Print and shaded views of the part. All mm, measured from the part's lowest x, y and z. Coordinates: 2 decimals unless noted, no trailing zeros. Order: outer loops, then holes, each group sorted by start corner. A loop starts at its lowest first (then second) coordinate and runs counter-clockwise, first axis right, second up. Notation, with made-up numbers: (-31.75, 44) - (-19.75, 44) arc R19 cw to (-19.75, 65) - close; hole circle Ø11 at (36, 54.25). An arc over 180 degrees is marked (long way). Write each question's results on one line, items separated by ' | '.
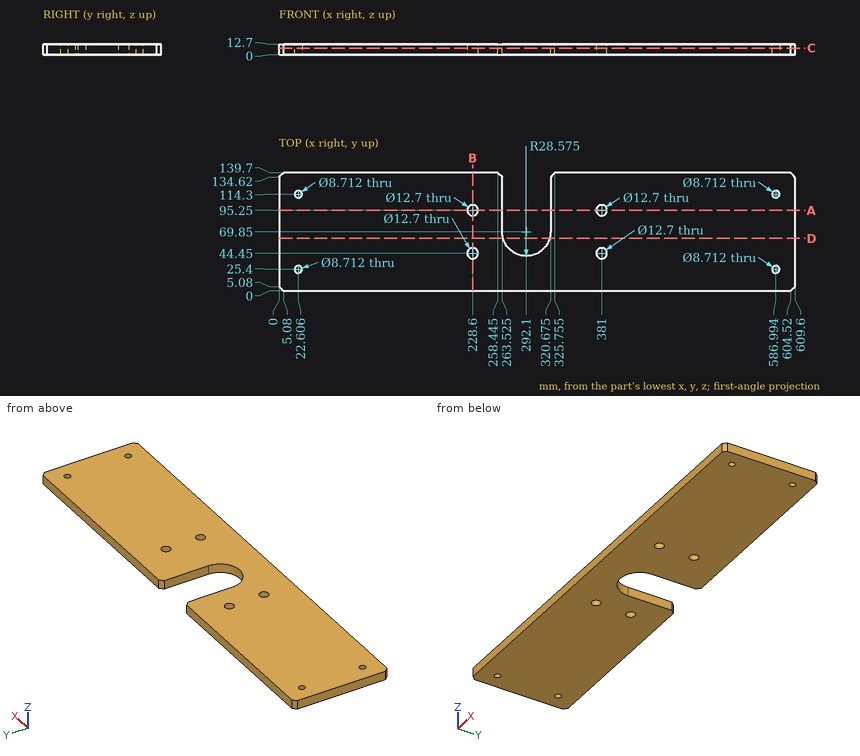
1. Band-saw the part on A-A on y = 95.25. Give the cut face in (x, z) (3 decimals), then the cut area to 3 significant figures.
Solved:
outline: (0, 0) - (222.25, 0) - (222.25, 12.7) - (0, 12.7) - close; (234.95, 0) - (263.525, 0) - (263.525, 12.7) - (234.95, 12.7) - close; (320.675, 0) - (374.65, 0) - (374.65, 12.7) - (320.675, 12.7) - close; (387.35, 0) - (609.6, 0) - (609.6, 12.7) - (387.35, 12.7) - close | area: 6,690 mm2
2. Band-saw the part on B-B on x = 228.6. Give the cut face in (y, z), then the cut area to 3 significant figures.
Solved:
outline: (0, 0) - (38.1, 0) - (38.1, 12.7) - (0, 12.7) - close; (50.8, 0) - (88.9, 0) - (88.9, 12.7) - (50.8, 12.7) - close; (101.6, 0) - (139.7, 0) - (139.7, 12.7) - (101.6, 12.7) - close | area: 1,450 mm2
3. Band-saw the part on C-C on z = 7.75. Give the number of separate pieces and of enclosed holes in the cut face, then the cut area to 3 significant figures.
Solved:
separate pieces: 1 | enclosed holes: 8 | area: 79,100 mm2
4. Drop flat-ended pins along their axis: pin 1 Ø7.5 at (x, y) = (381, 44.45) entering from -Z; pin 2 Ø1.5 at (x, z) = (307.5, 5.5) entering from +Y; pin 3 Ø3 at (x, z) = (262, 5) entering from +Y (1 decimal). Give the stop position or say it passes through.
Solved:
pin 1: passes through | pin 2: stops at y = 46.28 | pin 3: stops at y = 137.6
5. Probe line 1 (Y direction, x = 228.6, z = 10.25); line 2 (X direction, y = 76.5, z = 9.75) (3 decimals); line 3 (Y direction, x = 384, z = 11.25). List the from-to ranges inside material, lowest first.
Solved:
line 1: y = 0 to 38.1, 50.8 to 88.9, 101.6 to 139.7 | line 2: x = 0 to 263.525, 320.675 to 609.6 | line 3: y = 0 to 38.85, 50.05 to 89.65, 100.85 to 139.7
6. Band-saw the part on D-D on y = 62. Give the cut face in (x, z).
Solved:
outline: (0, 0) - (264.62, 0) - (264.62, 12.7) - (0, 12.7) - close; (319.58, 0) - (609.6, 0) - (609.6, 12.7) - (319.58, 12.7) - close
